from build123d import *

# Parameters (mm, degrees)
BOSS_EXTRUDE1_DEPTH      = 11
BOSS_EXTRUDE2_START      = 11
BOSS_EXTRUDE2_DEPTH      = 1
BOSS_EXTRUDE3_START      = 11
SKETCH5_W                = 5
SKETCH5_H                = 6
SKETCH5_W_2              = 6.5
BOSS_EXTRUDE3_DEPTH      = 7
SKETCH9_R                = 2.25
BOSS_EXTRUDE4_DEPTH      = 3
BOSS_EXTRUDE5_DEPTH      = 5
SKETCH7_R                = 1.75
TUBE_HOLES_DEPTH         = 4
PALM_TUBE_OPENING_DEPTH  = 10
WRIST_TUBE_OPENING_DEPTH = 5
SKETCH13_W               = 5
SKETCH13_H               = 6
SKETCH13_W_2             = 6.5
SKETCH13_H_2             = 7
CUT_EXTRUDE1_DEPTH       = 4
FILLET1_R                = 2
POT_INSERT_DEPTH         = 2.5
SCREW_START              = 12
SKETCH6_R                = 0.8
SCREW_HOLES_DEPTH        = 18
SKETCH10_R               = 1.25
SCREW_HEADS_DEPTH        = 2
CUT_EXTRUDE2_DEPTH       = 7
CUT_EXTRUDE4_DEPTH       = 7


with BuildPart() as part:
    # Sketch1 → Boss-Extrude1 (new body)
    with BuildSketch(Plane(origin=(0, 0, 0), x_dir=(1, 0, 0), z_dir=(0, 1, 0))):
        with BuildLine():
            Line((24.994192305, 10.517747211), (0.994192305, 10.517747211))
            Line((0.994192305, 10.517747211), (-0.899142434, 12.41108195))
            Line((-0.899142434, 12.41108195), (-5.848889902, 7.461334481))
            Line((-5.848889902, 7.461334481), (-17.86980821, 19.482252789))
            Line((-17.86980821, 19.482252789), (-28.348953445, 9.003107554))
            Line((-28.348953445, 9.003107554), (-34.005807695, 14.659961804))
            Line((-34.005807695, 14.659961804), (-34.005807695, 0.517747211))
            Line((-34.005807695, 0.517747211), (-29.005807695, -4.482252789))
            Line((-29.005807695, -4.482252789), (-29.005807695, -9.482252789))
            Line((-29.005807695, -9.482252789), (-12.005807695, -9.482252789))
            Line((-12.005807695, -9.482252789), (-12.005807695, -19.482252789))
            Line((-12.005807695, -19.482252789), (33.994192305, -19.482252789))
            Line((33.994192305, -19.482252789), (33.994192305, -15.482252791))
            Line((33.994192305, -15.482252791), (38.994192305, -15.482252791))
            Line((38.994192305, -15.482252791), (38.994192305, -9.482252791))
            Line((38.994192305, -9.482252791), (45.994192305, -9.482252791))
            Line((45.994192305, -9.482252791), (45.994192305, -15.482252791))
            Line((45.994192305, -15.482252791), (50.994192304, -15.482252791))
            Line((50.994192304, -15.482252791), (50.994192304, -4.314649764))
            ThreePointArc((50.994192304, -4.314649764), (36.049920395, -2.74875195), (28.994192305, 10.517747211))
            Line((28.994192305, 10.517747211), (24.994192305, 10.517747211))
        make_face()
        Polygon((13.494192305, -16.482252789), (32.994192305, -16.482252789), (32.994192305, -8.592903632), (24.994192305, -0.592903632), (24.994192305, 9.517747211), (1.864171021, 9.517747211), (-5.84899293, 1.80458326), (-19.991128553, 15.946718883), (-33.005807695, 2.932039742), (-33.005807695, 0.931960773), (-28.005807695, -4.068039227), (-28.005807695, -8.482252789), (-11.005807695, -8.482252789), (-11.005807695, -16.482252789), (8.494192305, -16.482252789), (8.494192305, -9.482252792), (13.494192305, -9.482252792), align=None, mode=Mode.SUBTRACT)
    extrude(amount=BOSS_EXTRUDE1_DEPTH)

    # Sketch3 → Boss-Extrude2 (add)
    with BuildSketch(Plane(origin=(0, 0, 0), x_dir=(1, 0, 0), z_dir=(0, 1, 0)).offset(BOSS_EXTRUDE2_START)):
        with BuildLine():
            Line((-17.86980821, 19.482252789), (-5.848889902, 7.461334481))
            Line((-5.848889902, 7.461334481), (-0.899142434, 12.41108195))
            Line((-0.899142434, 12.41108195), (0.994192305, 10.517747211))
            Line((0.994192305, 10.517747211), (24.994192305, 10.517747211))
            Line((24.994192305, 10.517747211), (28.994192305, 10.517747211))
            ThreePointArc((28.994192305, 10.517747211), (36.049920395, -2.74875195), (50.994192304, -4.314649764))
            Line((50.994192304, -4.314649764), (50.994192304, -15.482252791))
            Line((50.994192304, -15.482252791), (45.994192305, -15.482252791))
            Line((45.994192305, -15.482252791), (45.994192305, -9.482252791))
            Line((45.994192305, -9.482252791), (38.994192305, -9.482252791))
            Line((38.994192305, -9.482252791), (38.994192305, -15.482252791))
            Line((38.994192305, -15.482252791), (33.994192305, -15.482252791))
            Line((33.994192305, -15.482252791), (33.994192305, -19.482252789))
            Line((33.994192305, -19.482252789), (-12.005807695, -19.482252789))
            Line((-12.005807695, -19.482252789), (-12.005807695, -9.482252789))
            Line((-12.005807695, -9.482252789), (-29.005807695, -9.482252789))
            Line((-29.005807695, -9.482252789), (-29.005807695, -4.482252789))
            Line((-29.005807695, -4.482252789), (-34.005807695, 0.517747211))
            Line((-34.005807695, 0.517747211), (-34.005807695, 14.659961804))
            Line((-34.005807695, 14.659961804), (-28.348953445, 9.003107554))
            Line((-28.348953445, 9.003107554), (-17.86980821, 19.482252789))
        make_face()
    extrude(amount=-BOSS_EXTRUDE2_DEPTH)

    # Sketch5 → Boss-Extrude3 (add)
    with BuildSketch(Plane(origin=(0, 0, 0), x_dir=(1, 0, 0), z_dir=(0, 1, 0)).offset(BOSS_EXTRUDE3_START)):
        with Locations((-26.505807695, -12.482252789)):
            Rectangle(SKETCH5_W, SKETCH5_H)
        with Locations((-15.255807695, -12.482252789)):
            Rectangle(SKETCH5_W_2, SKETCH5_H)
    extrude(amount=-BOSS_EXTRUDE3_DEPTH)

    # Sketch9 → Boss-Extrude4 (add)
    with BuildSketch(Plane(origin=(0.80622229, 0, -0.80622229), x_dir=(-0.707106781, 0, -0.707106781), z_dir=(0.707106781, 0, -0.707106781))):
        with Locations((20.911895624, 0)):
            Circle(SKETCH9_R)
    extrude(amount=BOSS_EXTRUDE4_DEPTH)

    # Sketch11 → Boss-Extrude5 (add)
    with BuildSketch(Plane(origin=(0, 0, 0), x_dir=(1, 0, 0), z_dir=(0, 1, 0))):
        Polygon((-17.86980821, 19.482252789), (-20.698235335, 16.653825665), (-5.84899293, 1.80458326), (1.929181663, 9.582757853), (-0.899142434, 12.41108195), (-5.848889902, 7.461334481), align=None)
    extrude(amount=-BOSS_EXTRUDE5_DEPTH)

    # Sketch7 → Tube Holes (cut)
    with BuildSketch(Plane(origin=(-6.655112192, 0, -6.655112192), x_dir=(-0.707106781, 0, 0.707106781), z_dir=(-0.707106781, 0, -0.707106781))):
        with Locations((-4.640170496, 2)):
            Circle(SKETCH7_R)
        with Locations((-4.640170496, -2)):
            Circle(SKETCH7_R)
    extrude(amount=-TUBE_HOLES_DEPTH, mode=Mode.SUBTRACT)

    # Sketch8 → Palm Tube Opening (cut)
    with BuildSketch(Plane(origin=(0, 0, 0), x_dir=(1, 0, 0), z_dir=(0, 1, 0))):
        Polygon((24.994192305, 10.517747211), (0.994192305, 10.517747211), (1.929181663, 9.582757853), (1.864171021, 9.517747211), (27.864171021, -16.482252789), (32.994192305, -16.482252789), (32.994192305, -10.369554414), (28.931746465, -14.432000255), (20.044444837, -5.544698627), (24.994192305, -0.594951158), align=None)
        Polygon((-28.348953445, 9.003107554), (-20.698235335, 16.653825665), (-19.991128553, 15.946718883), (-27.641846664, 8.296000773), align=None)
    extrude(amount=PALM_TUBE_OPENING_DEPTH, mode=Mode.SUBTRACT)

    # Sketch12 → Wrist Tube Opening (cut)
    with BuildSketch(Plane(origin=(0, 0, 0), x_dir=(1, 0, 0), z_dir=(0, 1, 0))):
        Polygon((33.994192305, -19.482252789), (33.994192305, -9.592903632), (32.883541462, -8.482252789), (-12.005807695, -8.482252789), (-12.005807695, -19.482252789), align=None)
    extrude(amount=WRIST_TUBE_OPENING_DEPTH, mode=Mode.SUBTRACT)

    # Sketch13 → Cut-Extrude1 (cut)
    with BuildSketch(Plane(origin=(0, 0, 0), x_dir=(1, 0, 0), z_dir=(0, 1, 0))):
        with Locations((-26.505807695, -12.482252789)):
            Rectangle(SKETCH13_W, SKETCH13_H)
        with Locations((-15.255807695, -11.982252789)):
            Rectangle(SKETCH13_W_2, SKETCH13_H_2)
    extrude(amount=CUT_EXTRUDE1_DEPTH, mode=Mode.SUBTRACT)

    # Fillet1
    fillet1_edges = [part.edges().sort_by_distance(p)[0] for p in [
        (-34.005807695, 11, -7.588854507),
        (-31.505807695, 11, 1.982252789),
        (-29.005807695, 11, 9.982252789),
    ]]
    fillet(fillet1_edges, radius=FILLET1_R)

    # Sketch14 → Pot Insert (cut)
    with BuildSketch(Plane.ZY.offset(18.505807695)):
        Polygon((24.976594858, 1), (23.476594858, 4), (23.476594858, 5), (19.476594858, 5), (14.226594858, 5), (14.226594858, 4), (8.476594858, 4), (8.476594858, -0.5), (8.476594858, -5), (14.226594858, -5), (14.226594858, -6), (19.476594858, -6), (23.476594858, -6), (23.476594858, -5), (24.976594858, -2), (24.976594858, -0.5), align=None)
    extrude(amount=-POT_INSERT_DEPTH, mode=Mode.SUBTRACT)

    # Sketch6 → Screw Holes (cut, through all)
    with BuildSketch(Plane(origin=(0, 0, 0), x_dir=(1, 0, 0), z_dir=(0, 1, 0)).offset(SCREW_START)):
        with Locations((-31.141846664, 8.296000773)):
            Circle(SKETCH6_R)
        with Locations((-26.500149763, -10.976594858)):
            Circle(SKETCH6_R)
        with Locations((-26.500149763, -13.976594858)):
            Circle(SKETCH6_R)
        with Locations((-14.000149763, -13.976594858)):
            Circle(SKETCH6_R)
        with Locations((-14.000149763, -10.976594858)):
            Circle(SKETCH6_R)
        with Locations((10.994192305, -10.982252789)):
            Circle(SKETCH6_R)
        with Locations((10.994192305, -13.982252789)):
            Circle(SKETCH6_R)
        with Locations((-17.86980821, 16.653825665)):
            Circle(SKETCH6_R)
        with Locations((-5.84899293, 4.633010384)):
            Circle(SKETCH6_R)
        with Locations((27.316522776, 4.15378618)):
            Circle(SKETCH6_R)
        with Locations((38.630231275, -7.159922319)):
            Circle(SKETCH6_R)
        with Locations((36.494192305, -13.982252789)):
            Circle(SKETCH6_R)
        with Locations((36.494192305, -10.982252789)):
            Circle(SKETCH6_R)
        with Locations((48.494192305, -10.982252789)):
            Circle(SKETCH6_R)
        with Locations((48.494192305, -13.982252789)):
            Circle(SKETCH6_R)
    extrude(amount=-SCREW_HOLES_DEPTH, mode=Mode.SUBTRACT)

    # Sketch10 → Screw Heads (cut)
    with BuildSketch(Plane(origin=(0, 0, 0), x_dir=(1, 0, 0), z_dir=(0, 1, 0)).offset(SCREW_START)):
        with Locations((-17.86980821, 16.653825665)):
            Circle(SKETCH10_R)
        with Locations((-31.141846664, 8.296000773)):
            Circle(SKETCH10_R)
        with Locations((-26.500149763, -10.976594858)):
            Circle(SKETCH10_R)
        with Locations((-26.500149763, -13.976594858)):
            Circle(SKETCH10_R)
        with Locations((-14.000149763, -13.976594858)):
            Circle(SKETCH10_R)
        with Locations((-14.000149763, -10.976594858)):
            Circle(SKETCH10_R)
        with Locations((10.994192305, -10.982252789)):
            Circle(SKETCH10_R)
        with Locations((10.994192305, -13.982252789)):
            Circle(SKETCH10_R)
        with Locations((-5.84899293, 4.633010384)):
            Circle(SKETCH10_R)
        with Locations((27.316522776, 4.15378618)):
            Circle(SKETCH10_R)
        with Locations((38.630231275, -7.159922319)):
            Circle(SKETCH10_R)
        with Locations((36.494192305, -10.982252789)):
            Circle(SKETCH10_R)
        with Locations((36.494192305, -13.982252789)):
            Circle(SKETCH10_R)
        with Locations((48.494192305, -10.982252789)):
            Circle(SKETCH10_R)
        with Locations((48.494192305, -13.982252789)):
            Circle(SKETCH10_R)
    extrude(amount=-SCREW_HEADS_DEPTH, mode=Mode.SUBTRACT)

    # Sketch15 → Cut-Extrude2 (cut)
    with BuildSketch(Plane(origin=(0, 0, 0), x_dir=(1, 0, 0), z_dir=(0, 1, 0))):
        with BuildLine():
            Line((24.994192305, -0.592903632), (24.994192305, 10.517747211))
            Line((24.994192305, 10.517747211), (28.994192305, 10.517747211))
            ThreePointArc((28.994192305, 10.517747211), (36.049920395, -2.74875195), (50.994192304, -4.314649764))
            Line((50.994192304, -4.314649764), (50.994192304, -15.482252791))
            Line((50.994192304, -15.482252791), (45.994192305, -15.482252791))
            Line((45.994192305, -15.482252791), (45.994192305, -9.482252791))
            Line((45.994192305, -9.482252791), (38.994192305, -9.482252791))
            Line((38.994192305, -9.482252791), (38.994192305, -15.482252791))
            Line((38.994192305, -15.482252791), (33.994192305, -15.482252791))
            Line((33.994192305, -15.482252791), (33.994192305, -9.592903632))
            Line((33.994192305, -9.592903632), (24.994192305, -0.592903632))
        make_face()
    extrude(amount=CUT_EXTRUDE2_DEPTH, mode=Mode.SUBTRACT)

    # Sketch19 → Cut-Extrude4 (cut)
    with BuildSketch(Plane(origin=(12.200644337, 0, -12.200644337), x_dir=(0.707106781, 0, 0.707106781), z_dir=(-0.707106781, 0, 0.707106781))):
        with BuildLine():
            Line((19.878528118, 8.5), (19.878528118, 7))
            Line((19.878528118, 7), (28.878528118, 7))
            Line((28.878528118, 7), (28.878528118, 8.5))
            ThreePointArc((28.878528118, 8.5), (28.43918829, 9.560660172), (27.378528118, 10))
            Line((27.378528118, 10), (21.378528118, 10))
            ThreePointArc((21.378528118, 10), (20.317867946, 9.560660172), (19.878528118, 8.5))
        make_face()
    extrude(amount=-CUT_EXTRUDE4_DEPTH, mode=Mode.SUBTRACT)


solid = part.part
Could you check a few things on this model? Use its own coordinates, in mm. A direction names the side the tool comes from. Give positions to 0.01 mm unless a question says otherwise; leave off trailing zeros. Write each loop counter-clockwise with the first axis right and the second up, starting at its lowest first coordinate (ties: lowest second). Pieces come first, ordered by that corner, then holes. Notation, with made-up numbers: (-17, 14) -> (0, 14) arc R18 ccw to (0, 26) -> close; hole circle Ø7 at (49, -26). An arc over 180 degrees is marked (long way). Write each question's results on one line, items separated by ' | '. Start each with the question number.
Q1. Suppose I cut it at C-C, the plane x = 42.5. List the corners of the cut face in (y, z) for me, and give its area (3 significant figures).
Q2. Suppose I cut it at B-B, the plane y = 6. State how many separate pieces and enclosed holes the cut face has, and give its area (3 significant figures).
Q3. Which directions (+Z, -Z, +X, -X, +Y, -Y) give clear straight access to the entire face, cutting with the end or side of a thin tool? Please do faces 1 (the face through (28.89, 9.57, -0.14)), 2 (the face through (23, 7, 16.482)), 3 (the face through (38, 10, 8)), 4 (the face through (-18.506, 8, 13)).
Q4. I need wall thicknesses on probe 1 along X at (y, z) = (4.5, -9.5); probe 2 along Y at (x, z) = (26, 6); probe 3 along Z at (x, y) = (-5.5, -3). Which ranges of each line are inside material? Lowest first, please.
Q5. I'm going to push flat-ended pins straight in: pin 1 Ø6.5 at (y, z) = (6.5, 12) entering from -X; pin 2 Ø3 at (x, z) = (-14.5, 11) entering from +Y; pin 3 Ø1.8 at (x, z) = (-17.87, -16.65) entering from +Y; pin 4 Ø1.5 at (y, z) = (6, -14.5) entering from +X. Where does each tip first touch, or does it pass through?
Q6. We'd pull the mould along Z, two halves only. Please class faces 5 (the face through (27, 7, -6)), 6 (the face through (10.36, 7.54, 14.47)), 7 (the face through (19.2, 10.3, -10.518)): +Z half, -Z half, draft (parallel to the pull), parting line (faces both ways), or undercut.
Q7. Suppose I cut it at A-A, the plane x = 20. List the corners of the cut face in (y, z) for me, and give its area (3 significant figures).
Outcome:
1) outline: (7, 5.29) -> (11, 5.29) -> (11, 9.48) -> (7, 9.48) -> close | area: 16.8 mm2
2) separate pieces: 2 | enclosed holes: 9 | area: 422 mm2
3) face 1: +X, -Y | face 2: -Y | face 3: +Y | face 4: +Z, +Y, -Y
4) probe 1: -34.01 to -28.85, -13.54 to -7.89, -3.81 to 1.85 | probe 2: 10 to 11 | probe 3: -7.81 to -5.35, -3.91 to -2.15
5) pin 1: x = -29.01 | pin 2: y = 11 | pin 3: y = 10 | pin 4: x = -12.14
6) face 5: draft | face 6: undercut | face 7: -Z half
7) outline: (5, 16.48) -> (10, 16.48) -> (10, -10.52) -> (11, -10.52) -> (11, 19.48) -> (5, 19.48) -> close | area: 45.0 mm2
